Can you work these out from the drawing? Everything is in mm from the part's minimum corner. Coordinates: 2 decimals unless noted, no trailing zeros. Order: outer loops, then holes, each group sorted by start corner. A loop starts at its lowest first (then second) coordinate and runs counter-clockwise, first axis right, second up. Notation, with made-up numbers: (76.25, 68) - (132.25, 68) arc R25 ccw to (132.25, 82) - close; hole circle Ø3 at (26.25, -20.5). An arc over 180 degrees is marked (long way). Use a Markdown table: item, result. Add a question column.
(1) I want a section at A-A (x = 14). List the corners of the cut face in (y, z) for me.
(2) I want a section at C-C (y = 14). List the corners of the cut face in (x, z) for me.
(3) For pin 1 Ø3 at (y, z) = (17.5, 1) entering from -X; pin 2 Ø2.5 at (x, y) = (4.47, 8.5) entering from -Z; pin 3 Ø0.9 at (x, y) = (14.5, 25) entering from +Z, each with a flat end and sliding along its axis, tell me the tip position at first contact or that it passes through.
(4) I want a section at B-B (z = 0.4). List the corners of the cut face in (x, y) for me.
(5) I want a section at D-D (x = 11). List the corners of the cut face in (y, z) for me (1 decimal).
(6) If I drill on L1, parallel to Y at x = 17.75, z = 3.8; L2, parallel to Y at x = 14, z = 3.55, over which ranges is the centre line in solid material (lowest first)? Write a range as [from, to].
(7) We'd pull the mould along X, two halves only. Please class the marked faces 1, 2, 3 and 4: pulls with the +X half, pulls with the -X half, needs draft (parallel to the pull), parting line crosses it, or undercut.
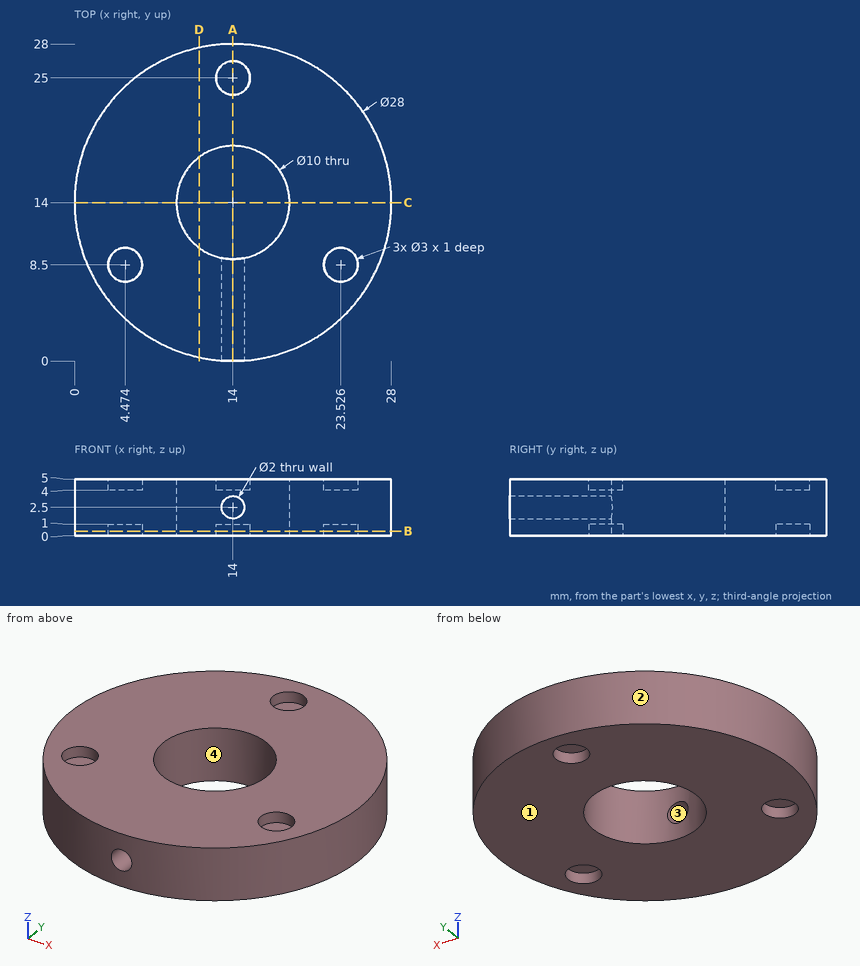
Answers follow:
| question | item | result |
|---|---|---|
| 1 | outline | (0, 0) - (9, 0) - (9, 1.5) - (0, 1.5) - close; (0, 3.5) - (9, 3.5) - (9, 5) - (0, 5) - close; (19, 0) - (23.5, 0) - (23.5, 1) - (26.5, 1) - (26.5, 0) - (28, 0) - (28, 5) - (26.5, 5) - (26.5, 4) - (23.5, 4) - (23.5, 5) - (19, 5) - close |
| 2 | outline | (0, 0) - (9, 0) - (9, 5) - (0, 5) - close; (19, 0) - (28, 0) - (28, 5) - (19, 5) - close |
| 3 | pin 1 | stops at x = 0.14 |
| 3 | pin 2 | stops at z = 1 |
| 3 | pin 3 | stops at z = 4 |
| 4 | outline | circle Ø28 at (14, 14); hole circle Ø3 at (4.47, 8.5); hole circle Ø10 at (14, 14); hole circle Ø3 at (14, 25); hole circle Ø3 at (23.53, 8.5) |
| 5 | outline | (0.3, 0) - (10, 0) - (10, 5) - (0.3, 5) - close; (18, 0) - (27.7, 0) - (27.7, 5) - (18, 5) - close |
| 6 | L1 | y = [0.51, 10.69], [17.31, 27.49] |
| 6 | L2 | y = [0, 9], [19, 28] |
| 7 | face 1 | needs draft |
| 7 | face 2 | parting line crosses it |
| 7 | face 3 | undercut |
| 7 | face 4 | undercut |
